```python
from build123d import *

# Parameters (mm, degrees)
BOSS_EXTRUDE1_START = 40
BOSS_EXTRUDE1_DEPTH = 2.5
SKETCH2_R           = 2.4
BOSS_EXTRUDE2_DEPTH = 22
CUT_EXTRUDE1_START  = 22
SKETCH2_3_R         = 1.5
CUT_EXTRUDE1_DEPTH  = 295.704277162
CHAMFER1_SIZE       = 2
CHAMFER1_SIZE2      = 5.494954839
CHAMFER2_SIZE       = 2
CHAMFER2_SIZE_2     = 5.494954839
SKETCH3_W           = 10
SKETCH3_H           = 5
BOSS_EXTRUDE3_DEPTH = 4.5
FILLET1_R           = 2
CUT_EXTRUDE2_REACH  = 287.714
SKETCH4_R           = 1.35
CUT_EXTRUDE3_REACH  = 293.869
SKETCH5_R           = 1.35
CUT_EXTRUDE4_REACH  = 188.832
SKETCH6_R           = 1.35
CUT_EXTRUDE5_REACH  = 188.762
SKETCH7_R           = 1.35


with BuildPart() as part:
    # Sketch1 → Boss-Extrude1 (new body)
    with BuildSketch(Plane.XZ.offset(-123.724152422).offset(BOSS_EXTRUDE1_START)):
        Polygon((7.812220157, 142.346117951), (14.049843919, 247.346117951), (106.533726398, 247.346117951), (112.70989627, 142.346117951), align=None)
    extrude(amount=BOSS_EXTRUDE1_DEPTH)

    # Sketch2 → Boss-Extrude2 (add)
    with BuildSketch(Plane(origin=(0, 83.724152422, 0), x_dir=(1, 0, 0), z_dir=(0, 1, 0))):
        with Locations(Location((36.196379089, -144.846126643, 0), (0, 0, 90))):
            Circle(SKETCH2_R)
        with Locations(Location((81.496379089, -144.846126643, 0), (0, 0, 90))):
            Circle(SKETCH2_R)
        with Locations(Location((31.696379089, -236.846126643, 0), (0, 0, 90))):
            Circle(SKETCH2_R)
        with Locations(Location((86.496379089, -206.846126643, 0), (0, 0, 90))):
            Circle(SKETCH2_R)
    extrude(amount=BOSS_EXTRUDE2_DEPTH)

    # Sketch2<3> → Cut-Extrude1 (cut, through all)
    with BuildSketch(Plane(origin=(0, 83.724152422, 0), x_dir=(1, 0, 0), z_dir=(0, 1, 0)).offset(CUT_EXTRUDE1_START)):
        with Locations(Location((81.496379089, -144.846126643, 0), (0, 0, 270))):
            Circle(SKETCH2_3_R)
        with Locations(Location((36.196379089, -144.846126643, 0), (0, 0, 270))):
            Circle(SKETCH2_3_R)
        with Locations(Location((86.496379089, -206.846126643, 0), (0, 0, 270))):
            Circle(SKETCH2_3_R)
        with Locations(Location((31.696379089, -236.846126643, 0), (0, 0, 270))):
            Circle(SKETCH2_3_R)
    extrude(amount=-CUT_EXTRUDE1_DEPTH, mode=Mode.SUBTRACT)

    # Chamfer1
    chamfer1_edges = [part.edges().sort_by_distance(p)[0] for p in [
        (86.496379089, 83.724152422, 209.246126643),
        (31.696379089, 83.724152422, 239.246126643),
    ]]
    chamfer1_side = [part.faces().sort_by_distance(p)[0] for p in [
        (60.285277184, 83.724152422, 193.81865211),
    ]]
    chamfer(chamfer1_edges, length=CHAMFER1_SIZE, length2=CHAMFER1_SIZE2, reference=chamfer1_side[0])

    # Chamfer2
    # the kernel refuses this chamfer: 5.494954839, 2 mm, written as the material it adds along each edge
    with BuildSketch(Plane(origin=(36.196379089, 83.724152422, 144.846126643), x_dir=(0, 0, -1), z_dir=(1, 0, 0))) as chamfer2_piece_1_section:
        Polygon((2.4 + CHAMFER2_SIZE, 0), (2.4, CHAMFER2_SIZE_2), (2.4, 0), align=None)
    chamfer2_piece_1 = revolve(axis=Axis((36.196379089, 83.724152422, 144.846126643), (0, 1, 0)), mode=Mode.PRIVATE)
    chamfer2_piece_1 = split(chamfer2_piece_1, bisect_by=Plane(origin=(36.196379089, 86.455650516, 142.346117951), z_dir=(0, 0, 1)), keep=Keep.TOP, mode=Mode.PRIVATE)
    add(chamfer2_piece_1)
    with BuildSketch(Plane(origin=(81.496379089, 83.724152422, 144.846126643), x_dir=(0, 0, -1), z_dir=(1, 0, 0))) as chamfer2_piece_2_section:
        Polygon((2.4 + CHAMFER2_SIZE, 0), (2.4, CHAMFER2_SIZE_2), (2.4, 0), align=None)
    chamfer2_piece_2 = revolve(axis=Axis((81.496379089, 83.724152422, 144.846126643), (0, 1, 0)), mode=Mode.PRIVATE)
    chamfer2_piece_2 = split(chamfer2_piece_2, bisect_by=Plane(origin=(81.496379089, 86.455650516, 142.346117951), z_dir=(0, 0, 1)), keep=Keep.TOP, mode=Mode.PRIVATE)
    add(chamfer2_piece_2)

    # Sketch3 → Boss-Extrude3 (add)
    with BuildSketch(Plane.XZ.offset(-81.224152422)):
        Polygon((12.267665701, 217.346117951), (17.861725107, 217.346117951), (17.861725107, 227.346117951), (12.861725107, 227.346117951), align=None)
        with Locations((25.262521401, 144.846117951)):
            Rectangle(SKETCH3_W, SKETCH3_H)
        Polygon((107.710131584, 227.318361744), (108.298338138, 217.318015768), (102.70427969, 217.321289832), (102.710132441, 227.321288119), align=None)
        Polygon((90.259589888, 142.328560554), (90.262516263, 147.328559698), (100.26251455, 147.322706947), (100.259588175, 142.322707804), align=None)
    extrude(amount=BOSS_EXTRUDE3_DEPTH)

    # Fillet1
    fillet1_edges = [part.edges().sort_by_distance(p)[0] for p in [
        (100.261051363, 76.724152422, 144.822707375),
        (95.262515407, 76.724152422, 147.325633323),
        (90.261053075, 76.724152422, 144.828560126),
        (20.262521401, 76.724152422, 144.846117951),
        (30.262521401, 76.724152422, 144.846117951),
        (25.262521401, 76.724152422, 147.346117951),
        (15.064695404, 76.724152422, 217.346117951),
        (17.861725107, 76.724152422, 222.346117951),
        (15.361725107, 76.724152422, 227.346117951),
        (105.210132013, 76.724152422, 227.319824931),
        (102.707206065, 76.724152422, 222.321288975),
        (105.501308914, 76.724152422, 217.3196528),
    ]]
    fillet(fillet1_edges, radius=FILLET1_R)

    # Sketch4 → Cut-Extrude2 (cut, up to next)
    with BuildSketch(Plane(origin=(120.663233846, 0, 7.097244942), x_dir=(0.05871713825649746, 0, -0.9982746604391837), z_dir=(0.9982746604391838, 0, 0.058717138256497464)), mode=Mode.PRIVATE) as cut_extrude2_sk1:
        with Locations((-215.601729693, 79.224152422)):
            Circle(SKETCH4_R)
    cut_extrude2_tool1 = extrude(cut_extrude2_sk1.sketch, amount=-CUT_EXTRUDE2_REACH, mode=Mode.PRIVATE) & part.part
    add(cut_extrude2_tool1.solids().sort_by_distance((108.003717, 79.224152, 222.326988))[0], mode=Mode.SUBTRACT)

    # Sketch5 → Cut-Extrude3 (cut, up to next)
    with BuildSketch(Plane(origin=(-0.641720197, 0, 0.038121992), x_dir=(0.05930139349204844, 0, 0.9982401237828007), z_dir=(-0.9982401237828007, 0, 0.05930139349204844)), mode=Mode.PRIVATE) as cut_extrude3_sk1:
        with Locations((222.691105358, 79.224152422)):
            Circle(SKETCH5_R)
    cut_extrude3_tool1 = extrude(cut_extrude3_sk1.sketch, amount=-CUT_EXTRUDE3_REACH, mode=Mode.PRIVATE) & part.part
    add(cut_extrude3_tool1.solids().sort_by_distance((12.564173, 79.224152, 222.337319))[0], mode=Mode.SUBTRACT)

    # Sketch6 → Cut-Extrude4 (cut, up to next)
    with BuildSketch(Plane(origin=(0, 0, 142.346117951), x_dir=(-1, 0, 0), z_dir=(0, 0, -1)), mode=Mode.PRIVATE) as cut_extrude4_sk1:
        with Locations((-25.262521401, 79.224152422)):
            Circle(SKETCH6_R)
    cut_extrude4_tool1 = extrude(cut_extrude4_sk1.sketch, amount=-CUT_EXTRUDE4_REACH, mode=Mode.PRIVATE) & part.part
    add(cut_extrude4_tool1.solids().sort_by_distance((25.262521, 79.224152, 142.346118))[0], mode=Mode.SUBTRACT)

    # Sketch7 → Cut-Extrude5 (cut, up to next)
    with BuildSketch(Plane(origin=(0.083332265, 0, 142.381338481), x_dir=(-0.9999998287265196, 0, 0.0005852750905060992), z_dir=(-0.0005852750905060992, 0, -0.9999998287265196)), mode=Mode.PRIVATE) as cut_extrude5_sk1:
        with Locations((-95.176273068, 79.224152422)):
            Circle(SKETCH7_R)
    cut_extrude5_tool1 = extrude(cut_extrude5_sk1.sketch, amount=-CUT_EXTRUDE5_REACH, mode=Mode.PRIVATE) & part.part
    add(cut_extrude5_tool1.solids().sort_by_distance((95.259589, 79.224152, 142.325634))[0], mode=Mode.SUBTRACT)


solid = part.part
```
Geometry check sheet. Reference: the model listing, model coordinates, mm. A direction names the side the tool comes from. Give positions to 0.01 mm unless a question says otherwise; leave off trailing zeros. Loops run counter-clockwise (first coordinate to the right, second up) from the corner with the lowest first, then second, coordinate; pieces in that order, holes last. Notation, with made-up numbers: M 0.5,6 L 43.5,6 A13 cw 43.5,29 Z; hole C -40,16.25 d9. An arc over 180 degrees is marked long. Write item = value, one per line. Start each with the question number.
1. Tool access check on faces 1 (the face through (20.263, 80, 145)), 2 (the face through (82.96, 97.36, 146.75)). Record the directions out of +Z, -Z, +X, -X, +Y, -Y that give a thin tool (end or side, any length) a straight path to the whole face; none if there is none.
2. Section check B-B, the plane x = 58. Enter the section's corners in (y, z), plus the area to 4 significant figures.
3. Section check C-C, the plane y = 97.5. Enter the section's corners in (x, z).
4. Draft check along X on faces 3 (the face through (24.64, 78.026, 144.811)), 4 (the face through (17.862, 81, 222)), 5 (the face through (107.935, 78.006, 223.499)), 6 (the face through (87.96, 97.36, 208.75)). Enter one of: +X half, -X half, draft (parallel to the pull), parting line (faces both ways), or undercut.
5. Go/stop test with flat-tipped pins: P1, Ø5, axis at x = 86.5, z = 206.85, coming from the -Y side; P2, Ø1.2, axis at x = 26, y = 80.5, coming from the +Z side; P3, Ø2, axis at y = 80, z = 222.5, coming from the +X side; P4, Ø1.5, axis at x = 30.5, y = 81, coming from the +Z side. Record where each tip stops, or that it passes through.
6. Thickness scan on probe 1 along Y at (x, z) = (70, 179); probe 2 along Z at (x, y) = (17, 83); probe 3 along X at (y, z) = (83, 198). Record the ranges inside material, lowest first.
7. Section check D-D, the plane z = 169. Enter the section's corners in (x, y).
8. Section check A-A, the plane y = 87.25. Enter the section's corners in (x, z), plus the area to 3 significant figures.
Values follow:
q1.face_1 = +Z, -Z, -X, -Y
q1.face_2 = +Y
q2.outline = M 81.22,142.35 L 83.72,142.35 L 83.72,247.35 L 81.22,247.35 Z
q2.area = 262.5 mm^2
q3.outline = C 31.7,236.85 d4.8; C 36.2,144.85 d4.8; C 81.5,144.85 d4.8; C 86.5,206.85 d4.8; hole C 31.7,236.85 d3; hole C 36.2,144.85 d3; hole C 81.5,144.85 d3; hole C 86.5,206.85 d3
q4.face_3 = undercut
q4.face_4 = undercut
q4.face_5 = +X half
q4.face_6 = parting line
q5.P1 = 81.22
q5.P2 = 147.35
q5.P3 = 108.05
q5.P4 = 247.35
q6.probe_1 = 81.22 to 83.72
q6.probe_2 = 142.35 to 247.35
q6.probe_3 = 11.12 to 109.44
q7.outline = M 9.4,81.22 L 111.14,81.22 L 111.14,83.72 L 9.4,83.72 Z
q8.outline = C 31.7,236.85 d6.23; M 34.34,142.35 L 38.06,142.35 A3.12 ccw long Z; M 79.64,142.35 L 83.36,142.35 A3.12 ccw long Z; C 86.5,206.85 d6.23; hole C 31.7,236.85 d3; hole C 36.2,144.85 d3; hole C 81.5,144.85 d3; hole C 86.5,206.85 d3
q8.area = 90.7 mm^2
